Part model, mm, in its own coordinate system. A direction names the side the tool comes from. Give positions to 0.01 mm unless a question says otherwise; leave off trailing zeros. Order: outer loops, then holes, each group sorted by start corner. A loop starts at its lowest first (then second) coordinate and runs counter-clockwise, first axis right, second up. Notation, with made-up numbers: (-5, 2) - (52, 2) arc R35 cw to (52, 36) - close; hole circle Ø5 at (19.25, 43.25). An arc over 180 degrees is marked (long way). One line per item, written item: value.
```python
from build123d import *

# Parameters (mm, degrees)
BOSS_EXTRUDE1_DEPTH = 25.4
SKETCH2_R           = 3.175
CUT_EXTRUDE1_DEPTH  = 41.40117325
SKETCH3_R           = 6.35
CUT_EXTRUDE2_DEPTH  = 2.54


with BuildPart() as part:
    # Sketch1 → Boss-Extrude1 (new body)
    with BuildSketch(Plane(origin=(0, 0, 0), x_dir=(0, 0, -1), z_dir=(1, 0, 0))):
        Polygon((27.94, 12.7), (30.48, 12.7), (30.48, 0), (0, 0), (0, 12.7), (2.54, 12.7), (2.54, 7.62), (27.94, 7.62), align=None)
    extrude(amount=BOSS_EXTRUDE1_DEPTH)

    # Sketch2 → Cut-Extrude1 (cut, through all)
    with BuildSketch(Plane(origin=(0, 7.62, 0), x_dir=(1, 0, 0), z_dir=(0, 1, 0))):
        with Locations(Location((12.7, 15.24, 0), (0, 0, 270))):
            Circle(SKETCH2_R)
    extrude(amount=-CUT_EXTRUDE1_DEPTH, mode=Mode.SUBTRACT)

    # Sketch3 → Cut-Extrude2 (cut)
    with BuildSketch(Plane(origin=(0, 7.62, 0), x_dir=(1, 0, 0), z_dir=(0, 1, 0))):
        with Locations(Location((12.7, 15.24, 0), (0, 0, 270))):
            Circle(SKETCH3_R)
    extrude(amount=-CUT_EXTRUDE2_DEPTH, mode=Mode.SUBTRACT)


solid = part.part
```
1) Pin check, flat tips, straight feed: pin 1 (14 mm diameter, centred on x = 11.5, z = -17.5, fed in from +Y); pin 2 (7.5 mm diameter, centred on x = 11.5, z = -13.5, fed in from +Y). Stop position of each tip, or through.
Outcome:
pin 1: stops at y = 7.62
pin 2: stops at y = 5.08
2) Cut at B-B, the plane x = 12.7. Give the cut face in (y, z) (3 decimals).
Outcome:
outline: (0, -30.48) - (12.7, -30.48) - (12.7, -27.94) - (7.62, -27.94) - (7.62, -21.59) - (5.08, -21.59) - (5.08, -18.415) - (0, -18.415) - close; (0, -12.065) - (5.08, -12.065) - (5.08, -8.89) - (7.62, -8.89) - (7.62, -2.54) - (12.7, -2.54) - (12.7, 0) - (0, 0) - close
3) Which spindle directions (+Z, -Z, +X, -X, +Y, -Y) get a long thin tool onto all of the face, cutting with end or side? Do faces 1 (the flat face through (13, 6, -30.48)), 2 (the flat face through (16, 5.08, -14)), 3 (the flat face through (10, 7.62, -9)). Say none if no direction does.
Outcome:
face 1: -Z, +X, -X, +Y, -Y
face 2: +Y
face 3: +X, -X, +Y
4) Mould opens along Z. For faces 4 (the flat face through (13, 10, -27.94)), 5 (the flat face through (25.4, 5, -15)), 6 (the flat face through (13, 6, 0)) say: released by +Z, released by -Z, zero draft, split by the parting line, or undercut.
Outcome:
face 4: undercut
face 5: zero draft
face 6: released by +Z
5) Cut at A-A, the plane z = -15.24. Give the cut face in (x, y) (3 decimals), then the cut area to 3 significant figures.
Outcome:
outline: (0, 0) - (9.525, 0) - (9.525, 5.08) - (6.35, 5.08) - (6.35, 7.62) - (0, 7.62) - close; (15.875, 0) - (25.4, 0) - (25.4, 7.62) - (19.05, 7.62) - (19.05, 5.08) - (15.875, 5.08) - close
area: 129 mm^2
6) Cut at D-D, the plane x = 4.5. Give the cut face in (y, z), then the cut area to 3 significant figures.
Outcome:
outline: (0, -30.48) - (12.7, -30.48) - (12.7, -27.94) - (7.62, -27.94) - (7.62, -2.54) - (12.7, -2.54) - (12.7, 0) - (0, 0) - close
area: 258 mm^2
7) Cut at C-C, the plane y = 6.5. Give the cut face in (x, z), then the cut area to 3 significant figures.
Outcome:
outline: (0, -30.48) - (25.4, -30.48) - (25.4, 0) - (0, 0) - close; hole circle Ø12.7 at (12.7, -15.24)
area: 648 mm^2
8) Drill centre lines: line 1 along X through (y, z) = (6.35, -15.24); line 2 along Z through (x, y) = (12.5, 9.75); line 3 along Y through (x, z) = (4.25, -15). Where is each one in solid material? Low to high. Write a range as from..to.
Outcome:
line 1: x = 0..6.35, 19.05..25.4
line 2: z = -30.48..-27.94, -2.54..0
line 3: y = 0..7.62
